Here's how the part is built. I have some questions about the finished solid (model axes, mm). A direction names the side the tool comes from. Round coordinates to 2 decimals unless told otherwise and drop trailing zeros. Loops run counter-clockwise (first coordinate to the right, second up) from the corner with the lowest first, then second, coordinate; pieces in that order, holes last. Notation, with made-up numbers: M 57,57 L 106,57 A20 ccw 106,63 Z; hole C 32,9.5 d8. An arc over 180 degrees is marked long. Answer as CSV lines item,"result".
```python
from build123d import *

# Parameters (mm, degrees)
SKETCH_1_W           = 52
SKETCH_1_H           = 14
EXTRUDE_1_DEPTH      = 11
SHELL_1_T            = -2
SKETCH_2_W           = 24
SKETCH_2_H           = 10
CUT_EXTRUDE_1_DEPTH  = 2
SKETCH_3_W           = 24
SKETCH_3_H           = 2
EXTRUDE_2_DEPTH      = 11
SKETCH_8_R           = 2
CUT_EXTRUDE_5_DEPTH  = 2
SKETCH_15_W          = 4
SKETCH_15_H          = 4
EXTRUDE_4_DEPTH      = 3
SKETCH_16_R          = 1.2
CUT_EXTRUDE_10_DEPTH = 10
FILLET_1_R           = 1
SKETCH_17_W          = 24
SKETCH_17_H          = 10
CUT_EXTRUDE_11_DEPTH = 1.6


with BuildPart() as part:
    # 草图1 → 凸台-拉伸1 (new body)
    with BuildSketch(Plane.XY):
        with Locations((26, 7)):
            Rectangle(SKETCH_1_W, SKETCH_1_H)
    extrude(amount=EXTRUDE_1_DEPTH)

    # 抽壳1
    shell_1_openings = [part.faces().sort_by_distance(p)[0] for p in [
        (26, 7, 0),
    ]]
    offset(amount=SHELL_1_T, openings=shell_1_openings, kind=Kind.INTERSECTION)

    # 草图2 → 切除-拉伸1 (cut)
    with BuildSketch(Plane(origin=(0, 0, 9), x_dir=(-1, 0, 0), z_dir=(0, 0, -1))):
        with Locations((-26, 7)):
            Rectangle(SKETCH_2_W, SKETCH_2_H)
    extrude(amount=-CUT_EXTRUDE_1_DEPTH, mode=Mode.SUBTRACT)

    # 草图3 → 凸台-拉伸2 (add)
    with BuildSketch(Plane.XY.offset(11)):
        with Locations((26, 1)):
            Rectangle(SKETCH_3_W, SKETCH_3_H)
        with Locations((26, 13)):
            Rectangle(SKETCH_3_W, SKETCH_3_H)
    extrude(amount=EXTRUDE_2_DEPTH)

    # 草图8 → 切除-拉伸5 (cut)
    with BuildSketch(Plane.XY.offset(11)):
        with Locations((8, 7)):
            Circle(SKETCH_8_R)
        with Locations((44, 7)):
            Circle(SKETCH_8_R)
    extrude(amount=-CUT_EXTRUDE_5_DEPTH, mode=Mode.SUBTRACT)

    # 草图15 → 凸台-拉伸4 (add)
    with BuildSketch(Plane.XY.offset(22)):
        with Locations((26, 4)):
            Rectangle(SKETCH_15_W, SKETCH_15_H)
        with Locations((26, 10)):
            Rectangle(SKETCH_15_W, SKETCH_15_H)
    extrude(amount=-EXTRUDE_4_DEPTH)

    # 草图19 → 切除-旋转6 (revolve, cut)
    with BuildSketch(Plane(origin=(0, 7, 0), x_dir=(1, 0, 0), z_dir=(0, 1, 0)), mode=Mode.PRIVATE) as cut_revolve_6_sk:
        Polygon((2.1, -11), (3.5, -11), (3.5, -9), (2.7, -9), (2.7, -9.9), align=None)
    revolve(cut_revolve_6_sk.sketch.rotate(Axis((3.5, 7, 11), (0, 0, -1)), 270), axis=Axis((3.5, 7, 11), (0, 0, -1)), mode=Mode.SUBTRACT)

    # 草图20 → 切除-旋转7 (revolve, cut)
    with BuildSketch(Plane(origin=(0, 7, 0), x_dir=(1, 0, 0), z_dir=(0, 1, 0)), mode=Mode.PRIVATE) as cut_revolve_7_sk:
        Polygon((11.1, -11), (12.5, -11), (12.5, -9), (11.7, -9), (11.7, -9.9), align=None)
    revolve(cut_revolve_7_sk.sketch.rotate(Axis((12.5, 7, 11), (0, 0, -1)), 270), axis=Axis((12.5, 7, 11), (0, 0, -1)), mode=Mode.SUBTRACT)

    # 草图21 → 切除-旋转8 (revolve, cut)
    with BuildSketch(Plane(origin=(0, 7, 0), x_dir=(1, 0, 0), z_dir=(0, 1, 0)), mode=Mode.PRIVATE) as cut_revolve_8_sk:
        Polygon((38.1, -11), (39.5, -11), (39.5, -9), (38.7, -9), (38.7, -9.9), align=None)
    revolve(cut_revolve_8_sk.sketch.rotate(Axis((39.5, 7, 11), (0, 0, -1)), 270), axis=Axis((39.5, 7, 11), (0, 0, -1)), mode=Mode.SUBTRACT)

    # 草图22 → 切除-旋转9 (revolve, cut)
    with BuildSketch(Plane(origin=(0, 7, 0), x_dir=(1, 0, 0), z_dir=(0, 1, 0)), mode=Mode.PRIVATE) as cut_revolve_9_sk:
        Polygon((47.1, -11), (48.5, -11), (48.5, -9), (47.7, -9), (47.7, -9.9), align=None)
    revolve(cut_revolve_9_sk.sketch.rotate(Axis((48.5, 7, 11), (0, 0, -1)), 270), axis=Axis((48.5, 7, 11), (0, 0, -1)), mode=Mode.SUBTRACT)

    # 草图16 → 切除-拉伸10 (cut)
    with BuildSketch(Plane.XY.offset(22)):
        with Locations((26, 10)):
            Circle(SKETCH_16_R)
        with Locations((26, 4)):
            Circle(SKETCH_16_R)
    extrude(amount=-CUT_EXTRUDE_10_DEPTH, mode=Mode.SUBTRACT)

    # 圆角1
    fillet_1_edges = [part.edges().sort_by_distance(p)[0] for p in [
        (52, 7, 11),
        (45, 14, 11),
        (45, 0, 11),
        (7, 14, 11),
        (38, 0, 16.5),
        (14, 0, 16.5),
        (0, 7, 11),
        (26, 14, 0),
        (14, 14, 16.5),
        (38, 14, 16.5),
        (52, 7, 0),
        (26, 0, 0),
        (0, 7, 0),
        (0, 14, 5.5),
        (52, 14, 5.5),
        (52, 0, 5.5),
        (0, 0, 5.5),
        (7, 0, 11),
    ]]
    fillet(fillet_1_edges, radius=FILLET_1_R)

    # 草图17 → 切除-拉伸11 (cut)
    with BuildSketch(Plane.XY.offset(22)):
        with Locations((26, 7)):
            Rectangle(SKETCH_17_W, SKETCH_17_H)
    extrude(amount=-CUT_EXTRUDE_11_DEPTH, mode=Mode.SUBTRACT)


solid = part.part
```
1. For P1, Ø3, axis at x = 26.5, y = 5, coming from the -Z side; P2, Ø1.1, axis at y = 1.5, z = 14.5, coming from the -X side; P3, Ø6, axis at x = 43.5, y = 7.5, coming from the +Z side; P4, Ø1, axis at x = 39.5, y = 7, coming from the +Z side, each with a flat end and sliding along its axis, tell me the tip position at first contact or that it passes through.
Evaluation:
P1,"stops at z = 19"
P2,"stops at x = 14"
P3,"stops at z = 11"
P4,"passes through"
2. We'd pull the mould along Y, two halves only. Please class faces 6 (the cylindrical face through (25.05, 9.27, 19.71)), 7 (the cylindrical face through (44.098, 0.285, 10.699)), 8 (the flat face through (6, 8, 11)): pulls with the +Y half, pulls with the -Y half, needs draft (parallel to the pull), parting line crosses it, or undercut.
Evaluation:
face 6,"undercut"
face 7,"pulls with the -Y half"
face 8,"needs draft"
3. I want a section at D-D, the plane z = 7.25. Please give me the cut outline in (x, y), and give its area (3 significant figures).
Evaluation:
outline,"M 0,1 A1 ccw 1,0 L 51,0 A1 ccw 52,1 L 52,13 A1 ccw 51,14 L 1,14 A1 ccw 0,13 Z; hole M 2,2 L 50,2 L 50,12 L 2,12 Z"
area,"247 mm²"
4. I want a section at A-A, the plane z = 15. Please give me the cut outline in (x, y).
Evaluation:
outline,"M 14,1 A1 ccw 15,0 L 37,0 A1 ccw 38,1 L 38,2 L 14,2 Z; M 14,12 L 38,12 L 38,13 A1 ccw 37,14 L 15,14 A1 ccw 14,13 Z"
5. I want a section at B-B, the plane x = 3.5. Please give me the cut outline in (y, z).
Evaluation:
outline,"M 0,1 A1 ccw 1,0 L 2,0 L 2,9 L 6.2,9 L 6.2,9.9 L 5.6,11 L 1,11 A1 ccw 0,10 Z; M 7.8,9 L 12,9 L 12,0 L 13,0 A1 ccw 14,1 L 14,10 A1 ccw 13,11 L 8.4,11 L 7.8,9.9 Z"
6. I want a section at C-C, the plane y = 10. Please give me the cut outline in (x, z).
Evaluation:
outline,"M 0,1 A1 ccw 1,0 L 2,0 L 2,9 L 14,9 L 14,11 L 1,11 A1 ccw 0,10 Z; M 24,19 L 24.8,19 L 24.8,20.4 L 24,20.4 Z; M 27.2,19 L 28,19 L 28,20.4 L 27.2,20.4 Z; M 38,9 L 50,9 L 50,0 L 51,0 A1 ccw 52,1 L 52,10 A1 ccw 51,11 L 38,11 Z"
7. Which directions (+Z, -Z, +X, -X, +Y, -Y) give clear straight access to the entire face, cutting with the end or side of a thin tool? Please do faces 1 (the flat face through (25, 11, 20.4)), 2 (the flat face through (14, 12.5, 16.4)), 3 (the cylindrical face through (37.699, 13.715, 16.084)), 4 (the cylindrical face through (8.098, 13.699, 10.715)), 5 (the flat face through (24, 10, 20)).
Evaluation:
face 1,"+Z, +X, -X"
face 2,"+Z, -X, +Y, -Y"
face 3,"+Z, +X, +Y"
face 4,"+Z, -X, +Y"
face 5,"+Z, -Z, -X"
8. If I drill on line 1 (Y direction, x = 26, z = 19.95); line 2 (Y direction, x = 23, z = 2.5); line 3 (Y direction, x = 44, z = 9.4), over which ranges is the centre line in solid material (lowest first)? Write a range as [from, to].
Evaluation:
line 1,"y = [0, 2.8], [5.2, 6], [8, 8.8], [11.2, 14]"
line 2,"y = [0, 2], [12, 14]"
line 3,"y = [0, 5], [9, 14]"
